Part print with two shaded views. Sizes in mm from the minimum x, y, z corner. Round coordinates to 2 decimals unless told otherwise and drop trailing zeros. Loops run counter-clockwise (first coordinate to the right, second up) from the corner with the lowest first, then second, coordinate; pieces in that order, holes last. Notation, with made-up numbers: M 18,48.5 L 72,48.5 A37 ccw 72,85.5 Z; hole C -9.75,-37.5 d7. An arc over 180 degrees is marked long. Use a Markdown table: item, result. Add a question column.
Item 1: Saw through at A-A on z = 9. Write the cut outline in (x, y).
Item 2: Two-plate mould, pull along X, no slides. Class the marked faces 1, 2 and 3: +X half, -X half, draft (parallel to the pull), parting line (faces both ways), or undercut.
Item 3: Wall check: L1, parallel to Z at x = 9, y = 3.8; L2, parallel to X at y = 1.4, z = 10; L3, parallel to Z at x = 2, y = 3.4. Give the ranges that are in metal, low to high. Write a range as from..to.
Item 4: Saw through at D-D on y = 0.4. Write the cut outline in (x, z), then the cut area to 3 significant figures.
Item 5: Pin check, flat tip, straight feed: P1, Ø1.4, axis at x = 2, z = 9, coming from the +Y side. Stop position of the tip, or through.
Item 6: Saw through at C-C on x = 2. Write the cut outline in (y, z).
Item 7: Saw through at B-B on x = 9. Write the cut outline in (y, z), then the cut area to 3 significant figures.
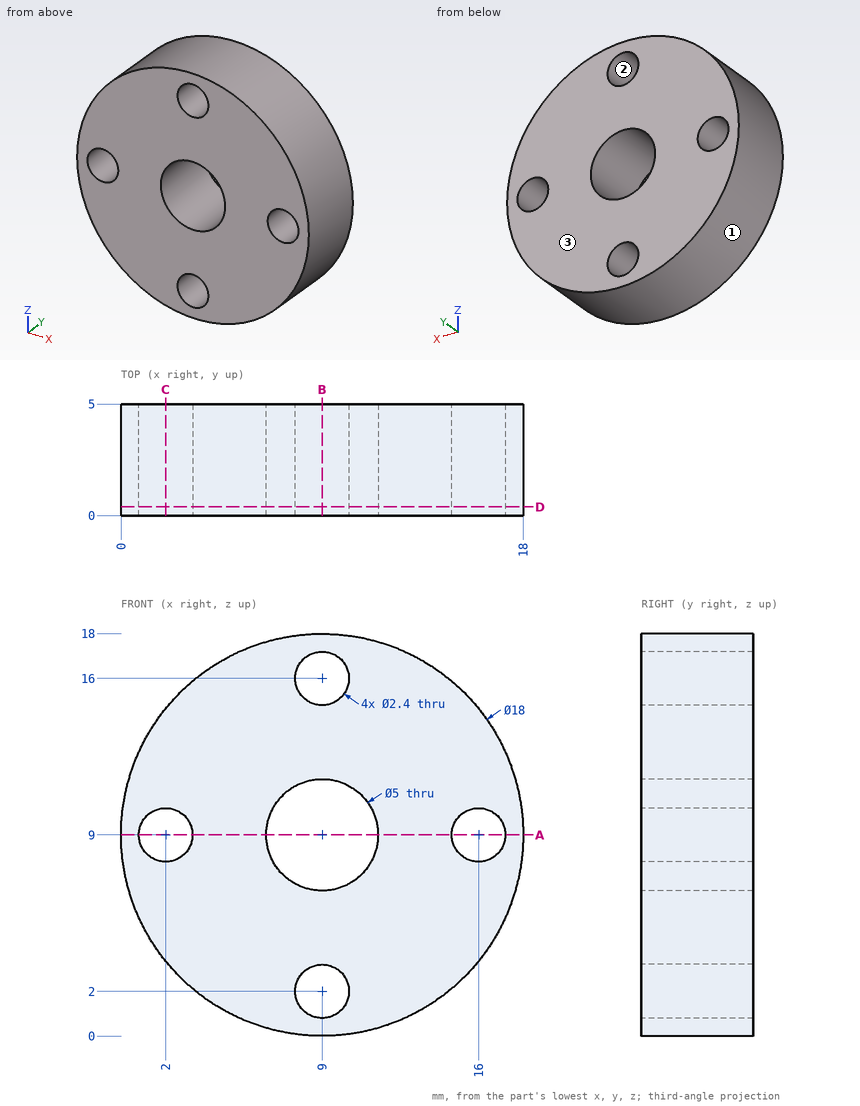
Entries:
| question | item | result |
|---|---|---|
| 1 | outline | M 0,0 L 0.8,0 L 0.8,5 L 0,5 Z; M 3.2,0 L 6.5,0 L 6.5,5 L 3.2,5 Z; M 11.5,0 L 14.8,0 L 14.8,5 L 11.5,5 Z; M 17.2,0 L 18,0 L 18,5 L 17.2,5 Z |
| 2 | face 1 | parting line |
| 2 | face 2 | undercut |
| 2 | face 3 | draft |
| 3 | L1 | 0..0.8, 3.2..6.5, 11.5..14.8, 17.2..18 |
| 3 | L2 | 0.06..1.34, 2.66..6.71, 11.29..15.34, 16.66..17.94 |
| 3 | L3 | 3.34..7.8, 10.2..14.66 |
| 4 | outline | C 9,9 d18; hole C 2,9 d2.4; hole C 9,9 d5; hole C 9,2 d2.4; hole C 9,16 d2.4; hole C 16,9 d2.4 |
| 4 | area | 217 mm2 |
| 5 | P1 | through |
| 6 | outline | M 0,3.34 L 5,3.34 L 5,7.8 L 0,7.8 Z; M 0,10.2 L 5,10.2 L 5,14.66 L 0,14.66 Z |
| 7 | outline | M 0,0 L 5,0 L 5,0.8 L 0,0.8 Z; M 0,3.2 L 5,3.2 L 5,6.5 L 0,6.5 Z; M 0,11.5 L 5,11.5 L 5,14.8 L 0,14.8 Z; M 0,17.2 L 5,17.2 L 5,18 L 0,18 Z |
| 7 | area | 41.0 mm2 |
